Here's how the part is built. I have some questions about the finished solid (model axes, mm). Face numbers are marked on the shaded views. A direction names the side the tool comes from. Give positions to 0.01 mm unless a question says otherwise; leave off trailing zeros. Loops run counter-clockwise (first coordinate to the right, second up) from the corner with the lowest first, then second, coordinate; pieces in that order, holes last.
Q1. Suppose I cut it at B-B (x = -1). List the corners of the cut face in (y, z) for me, and give its area (3 significant figures).
Q2. I'm going to push flat-ended pins straight in: P1, Ø3, axis at x = -21, z = -24.5, coming from the -Y side; P2, Ø2.5, axis at x = 21.69, z = -25.19, coming from the +Y side; P3, Ø1, axis at x = 8, z = -13.5, coming from the +Y side; P4, Ø6, axis at x = -4, y = -5.5, coming from the -Z side. Where does each tip first touch, or does it pass through?
Q3. For the marked faces 4, 5 and 6, which set-ups out of +Z, -Z, +X, -X, +Y, -Y let a thin tool reach every point of the face, with its end or its side?
Q4. Suppose I cut it at D-D (z = -18.84). List the corners of the cut face in (x, y) for me.
Q5. Thinking about a two-plate mould opening in X: for the marked faces 1, 2 and 3, which applies, pulls with the +X half, pulls with the -X half, needs draft (parallel to the pull), parting line crosses it, or undercut?
Q6. I need wall thicknesses on probe 1 along Z at (x, y) = (21.69, -19); probe 2 along Z at (x, y) = (-16, -7.5); probe 3 along Z at (x, y) = (23, -19). Which ranges of each line are inside material? Lowest first, please.
Q7. Suppose I cut it at A-A (y = -7). List the corners of the cut face in (x, z) for me.
Q8. Suppose I cut it at C-C (x = -21.69). List the corners of the cut face in (y, z) for me.
```python
from build123d import *

# Parameters (mm, degrees)
BOSS_EXTRUDE1_DEPTH = 24.500000006
SKETCH2_W           = 51
SKETCH2_H           = 38.1
SKETCH2_R           = 6.25
SKETCH2_R_2         = 1.7
BOSS_EXTRUDE2_DEPTH = 5
BOSS_EXTRUDE3_DEPTH = 29
SKETCH4_R           = 2.000000064
CUT_EXTRUDE1_DEPTH  = 6.99999997
SKETCH5_R           = 2.000000064
CUT_EXTRUDE2_DEPTH  = 6.99999997
CUT_EXTRUDE3_START  = -6.99999997
SKETCH6_R           = 2.000000064
CUT_EXTRUDE3_DEPTH  = 6.99999997


with BuildPart() as part:
    # Sketch1 → Boss-Extrude1 (new body)
    with BuildSketch(Plane.XY):
        with BuildLine():
            Line((18.5, 0), (25.5, 0))
            Line((25.5, 0), (25.5, -20.716))
            Line((25.5, -20.716), (-25.5, -20.716))
            Line((-25.5, -20.716), (-25.5, 0))
            Line((-25.5, 0), (-18.5, 0))
            ThreePointArc((-18.5, 0), (0, -18.5), (18.5, 0))
        make_face()
    extrude(amount=BOSS_EXTRUDE1_DEPTH)

    # Sketch2 → Boss-Extrude2 (add)
    with BuildSketch(Plane.XY.offset(24.500000006)):
        with Locations((0, -1.666)):
            Rectangle(SKETCH2_W, SKETCH2_H)
        with Locations((0, -7)):
            Circle(SKETCH2_R, mode=Mode.SUBTRACT)
        with Locations((15.5, 0)):
            Circle(SKETCH2_R_2, mode=Mode.SUBTRACT)
        with Locations((-7.75, -13.423393759)):
            Circle(SKETCH2_R_2, mode=Mode.SUBTRACT)
        with Locations((-7.75, 13.423393759)):
            Circle(SKETCH2_R_2, mode=Mode.SUBTRACT)
        with Locations((-15.5, 0)):
            Circle(SKETCH2_R_2, mode=Mode.SUBTRACT)
        with Locations((7.75, 13.423393759)):
            Circle(SKETCH2_R_2, mode=Mode.SUBTRACT)
        with Locations((7.75, -13.423393759)):
            Circle(SKETCH2_R_2, mode=Mode.SUBTRACT)
    extrude(amount=BOSS_EXTRUDE2_DEPTH)

    # Sketch3 → Boss-Extrude3 (add)
    with BuildSketch(Plane(origin=(0, 0, 0), x_dir=(-1, 0, 0), z_dir=(0, 0, -1))):
        with BuildLine():
            Line((16.75, 0), (25.5, 0))
            Line((25.5, 0), (25.5, -20.716))
            Line((25.5, -20.716), (-25.5, -20.716))
            Line((-25.5, -20.716), (-25.5, 0))
            Line((-25.5, 0), (-16.75, 0))
            ThreePointArc((-16.75, 0), (0, -16.75), (16.75, 0))
        make_face()
    extrude(amount=BOSS_EXTRUDE3_DEPTH)

    # Sketch4 → Cut-Extrude1 (cut)
    with BuildSketch(Plane.XZ.offset(20.716)):
        with Locations((-21.69, 25.690000006)):
            Circle(SKETCH4_R)
        with Locations((21.69, 25.690000006)):
            Circle(SKETCH4_R)
        with Locations((-21.69, -25.19)):
            Circle(SKETCH4_R)
        with Locations((21.69, -25.19)):
            Circle(SKETCH4_R)
    extrude(amount=-CUT_EXTRUDE1_DEPTH, mode=Mode.SUBTRACT)

    # Sketch5 → Cut-Extrude2 (cut)
    with BuildSketch(Plane.ZY.offset(25.5)):
        with Locations((-18.84, -15.636)):
            Circle(SKETCH5_R)
    extrude(amount=-CUT_EXTRUDE2_DEPTH, mode=Mode.SUBTRACT)

    # Sketch6 → Cut-Extrude3 (cut)
    with BuildSketch(Plane(origin=(25.5, 0, 0), x_dir=(0, 0, -1), z_dir=(1, 0, 0)).offset(CUT_EXTRUDE3_START)):
        with Locations(Location((18.84, -15.636, 0), (0, 0, 180))):
            Circle(SKETCH6_R)
    extrude(amount=CUT_EXTRUDE3_DEPTH, mode=Mode.SUBTRACT)


solid = part.part
```
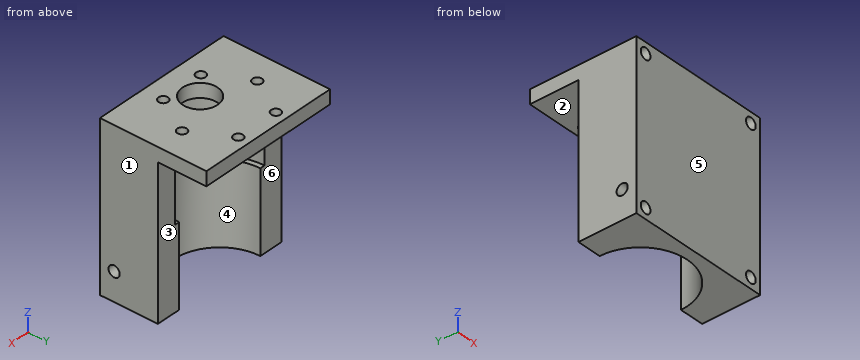
Solutions:
1. outline: (-20.72, -29) - (-16.72, -29) - (-16.72, 0) - (-18.47, 0) - (-18.47, 24.5) - (-13.17, 24.5) - (-13.17, 29.5) - (-20.72, 29.5) - close; (-0.83, 24.5) - (17.38, 24.5) - (17.38, 29.5) - (-0.83, 29.5) - close
1. area: 300 mm2
2. P1: stops at y = -20.72
2. P2: stops at y = 0
2. P3: stops at y = -14.43
2. P4: stops at z = 24.5
3. face 4: -Z, +Y
3. face 5: +Z, -Z, +X, -X, -Y
3. face 6: -Z, +X, -X, +Y
4. outline: (-25.5, -20.72) - (25.5, -20.72) - (25.5, -17.64) - (18.5, -17.64) - (18.5, -13.64) - (25.5, -13.64) - (25.5, 0) - (16.75, 0) arc R16.75 cw to (-16.75, 0) - (-25.5, 0) - (-25.5, -13.64) - (-18.5, -13.64) - (-18.5, -17.64) - (-25.5, -17.64) - close
5. face 1: pulls with the +X half
5. face 2: undercut
5. face 3: needs draft
6. probe 1: z = -29 to -27.19, -23.19 to 23.69, 27.69 to 29.5
6. probe 2: z = -29 to 0, 24.5 to 29.5
6. probe 3: z = -29 to -26.7, -23.68 to 24.18, 27.2 to 29.5
7. outline: (-25.5, -29) - (-15.22, -29) - (-15.22, 0) - (-17.12, 0) - (-17.12, 24.5) - (-6.25, 24.5) - (-6.25, 29.5) - (-25.5, 29.5) - close; (6.25, 24.5) - (17.12, 24.5) - (17.12, 0) - (15.22, 0) - (15.22, -29) - (25.5, -29) - (25.5, 29.5) - (6.25, 29.5) - close
8. outline: (-20.72, -29) - (0, -29) - (0, 24.5) - (17.38, 24.5) - (17.38, 29.5) - (-20.72, 29.5) - (-20.72, 27.69) - (-13.72, 27.69) - (-13.72, 23.69) - (-20.72, 23.69) - (-20.72, -23.19) - (-13.72, -23.19) - (-13.72, -27.19) - (-20.72, -27.19) - close; hole circle Ø4 at (-15.64, -18.84)
